Check sheet for the modelled part. Datum: model origin and axes. Units: mm. Face numbers are marked on the shaded views. Round coordinates to 2 decimals unless told otherwise and drop trailing zeros. Loops run counter-clockwise (first coordinate to the right, second up) from the corner with the lowest first, then second, coordinate; pieces in that order, holes last. Notation, with made-up numbers: (-20.5, 30.25) -> (4.5, 30.25) arc R19 ccw to (4.5, 34.25) -> close; hole circle Ø1 at (-38.5, 1.5). An arc over 180 degrees is marked (long way). Use one line per item in the form item = value. Start each with the question number.
(1) Draft check along Z on the marked faces 1, 2 and 3. Enter one of: released by +Z, released by -Z, zero draft, split by the parting line, or undercut.
(2) Sectioned sample at A-A (z = 14). Record the cut outline in (x, y).
(3) Go/stop test with flat-tipped pins: pin 1 (4 mm diameter, centred on x = 32.5, z = 30.5, fed in from +Y); pin 2 (2 mm diameter, centred on x = -75, z = 36.5, fed in from +Y); pin 3 (2 mm diameter, centred on x = 53.5, y = 11.5, fed in from -Z). Record where each tip stops, or that it passes through.
(4) Material ranges on probe 1 along X at (y, z) = (11.75, 36); probe 2 along Z at (x, y) = (-75, 5.5); probe 3 along Z at (x, y) = (-75, 13.5), recorded low to high. Write a range as [from, to].
(5) Sectioned sample at B-B (y = 7.5). State how many separate pieces and enclosed holes the cut face has, and give its area (3 significant figures).
(6) Sectioned sample at D-D (z = -9.5). Record the cut outline in (x, y).
(7) Sectioned sample at C-C (x = -16). Record the cut outline in (y, z).
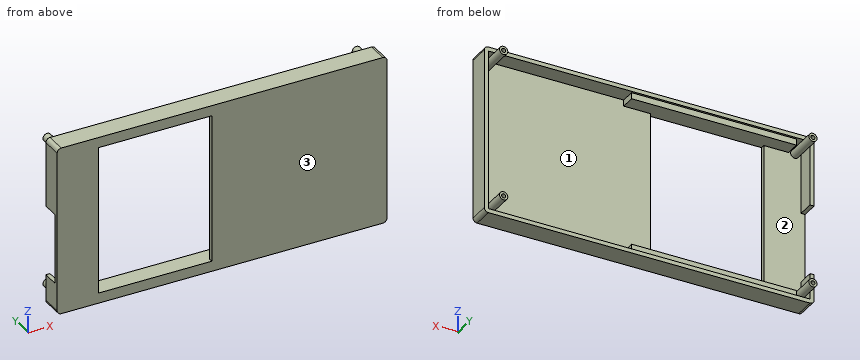
from build123d import *

# Parameters (mm, degrees)
SKETCH1_W           = 160
SKETCH1_H           = 82
BOSS_EXTRUDE1_DEPTH = 10
SHELL1_T            = -2
FILLET1_R           = 2
FILLET2_R           = 2
FILLET3_R           = 2
FILLET4_R           = 2
SKETCH10_W          = 34
SKETCH10_H          = 8.029729716
CUT_EXTRUDE1_DEPTH  = 6
SKETCH2_R           = 2
SKETCH2_R_2         = 1
BOSS_EXTRUDE7_DEPTH = 16
SKETCH12_W          = 80
SKETCH12_H          = 3
BOSS_EXTRUDE8_DEPTH = 7
SKETCH13_W          = 55
SKETCH13_H          = 72
CUT_EXTRUDE3_DEPTH  = 200


with BuildPart() as part:
    # Sketch1 → Boss-Extrude1 (new body)
    with BuildSketch(Plane(origin=(0, 0, 0), x_dir=(1, 0, 0), z_dir=(0, 1, 0))):
        Rectangle(SKETCH1_W, SKETCH1_H)
    extrude(amount=BOSS_EXTRUDE1_DEPTH)

    # Shell1
    shell1_openings = [part.faces().sort_by_distance(p)[0] for p in [
        (0, 10, 0),
    ]]
    offset(amount=SHELL1_T, openings=shell1_openings, kind=Kind.INTERSECTION)

    # Fillet1
    fillet1_edges = [part.edges().sort_by_distance(p)[0] for p in [
        (-80, 5, 41),
    ]]
    fillet(fillet1_edges, radius=FILLET1_R)

    # Fillet2
    fillet2_edges = [part.edges().sort_by_distance(p)[0] for p in [
        (-80, 5, -41),
    ]]
    fillet(fillet2_edges, radius=FILLET2_R)

    # Fillet3
    fillet3_edges = [part.edges().sort_by_distance(p)[0] for p in [
        (80, 5, -41),
    ]]
    fillet(fillet3_edges, radius=FILLET3_R)

    # Fillet4
    fillet4_edges = [part.edges().sort_by_distance(p)[0] for p in [
        (80, 5, 41),
    ]]
    fillet(fillet4_edges, radius=FILLET4_R)

    # Sketch10 → Cut-Extrude1 (cut)
    with BuildSketch(Plane.ZY.offset(80)):
        with Locations((-9.4, 6.014864858)):
            Rectangle(SKETCH10_W, SKETCH10_H)
    extrude(amount=-CUT_EXTRUDE1_DEPTH, mode=Mode.SUBTRACT)

    # Sketch2 → Boss-Extrude7 (add)
    # profile 1 of 4: a face of its own
    with BuildSketch(Plane(origin=(0, 2, 0), x_dir=(1, 0, 0), z_dir=(0, 1, 0))):
        with Locations(Location((-75, 36, 0), (0, 0, 90))):
            Circle(SKETCH2_R)
        with Locations(Location((-75, 36, 0), (0, 0, 270))):
            Circle(SKETCH2_R_2, mode=Mode.SUBTRACT)
    # profile 2 of 4: a face of its own
    with BuildSketch(Plane(origin=(0, 2, 0), x_dir=(1, 0, 0), z_dir=(0, 1, 0))):
        with Locations(Location((75, 36, 0), (0, 0, 90))):
            Circle(SKETCH2_R)
        with Locations(Location((75, 36, 0), (0, 0, 90))):
            Circle(SKETCH2_R_2, mode=Mode.SUBTRACT)
    # profile 3 of 4: a face of its own
    with BuildSketch(Plane(origin=(0, 2, 0), x_dir=(1, 0, 0), z_dir=(0, 1, 0))):
        with Locations(Location((-75, -36, 0), (0, 0, 90))):
            Circle(SKETCH2_R)
        with Locations(Location((-75, -36, 0), (0, 0, 90))):
            Circle(SKETCH2_R_2, mode=Mode.SUBTRACT)
    # profile 4 of 4: a face of its own
    with BuildSketch(Plane(origin=(0, 2, 0), x_dir=(1, 0, 0), z_dir=(0, 1, 0))):
        with Locations(Location((75, -36, 0), (0, 0, 90))):
            Circle(SKETCH2_R)
        with Locations(Location((75, -36, 0), (0, 0, 270))):
            Circle(SKETCH2_R_2, mode=Mode.SUBTRACT)
    extrude(amount=BOSS_EXTRUDE7_DEPTH)

    # Sketch12 → Boss-Extrude8 (add)
    with BuildSketch(Plane(origin=(0, 2, 0), x_dir=(1, 0, 0), z_dir=(0, 1, 0))):
        with Locations((-32, 37.5)):
            Rectangle(SKETCH12_W, SKETCH12_H)
        with Locations((-32, -37.5)):
            Rectangle(SKETCH12_W, SKETCH12_H)
    extrude(amount=BOSS_EXTRUDE8_DEPTH)

    # Sketch13 → Cut-Extrude3 (cut)
    with BuildSketch(Plane(origin=(0, 2, 0), x_dir=(1, 0, 0), z_dir=(0, 1, 0))):
        with Locations((-32.5, 0)):
            Rectangle(SKETCH13_W, SKETCH13_H)
    extrude(amount=-CUT_EXTRUDE3_DEPTH, mode=Mode.SUBTRACT)


solid = part.part
Checks:
q1.face_1 = undercut
q1.face_2 = undercut
q1.face_3 = zero draft
q2.outline = (-80, 0) -> (-60, 0) -> (-60, 2) -> (-78, 2) -> (-78, 10) -> (-80, 10) -> close; (-5, 0) -> (80, 0) -> (80, 10) -> (78, 10) -> (78, 2) -> (-5, 2) -> close
q3.pin_1 = 2
q3.pin_2 = 18
q3.pin_3 = through
q4.probe_1 = [-77, -76], [-74, -73], [73, 74], [76, 77]
q4.probe_2 = [-41, -39], [-38, -37], [-35, -34], [34, 35], [37, 38], [39, 41]
q4.probe_3 = [-38, -37], [-35, -34], [34, 35], [37, 38]
q5.separate_pieces = 5
q5.enclosed_holes = 4
q5.area = 1,400 mm2
q6.outline = (-80, 0) -> (-60, 0) -> (-60, 2) -> (-80, 2) -> close; (-5, 0) -> (80, 0) -> (80, 10) -> (78, 10) -> (78, 2) -> (-5, 2) -> close
q7.outline = (0, -41) -> (10, -41) -> (10, -39) -> (9, -39) -> (9, -36) -> (0, -36) -> close; (0, 36) -> (9, 36) -> (9, 39) -> (10, 39) -> (10, 41) -> (0, 41) -> close
